Design review of the part shown in the three views and the two pictorial views. Dimensions are in mm from the part's minimum x, y and z. A direction names the side the tool comes from. Give positions to 0.01 mm unless a question says otherwise; leave off trailing zeros. Loops run counter-clockwise (first coordinate to the right, second up) from the corner with the lowest first, then second, coordinate; pieces in that order, holes last. Notation, with made-up numbers: (62, 25.5) - (71, 25.5) arc R20 cw to (71, 37.5) - close; hole circle Ø6 at (40.25, 3). An arc over 180 degrees is marked (long way). Put each result on its own line as item: value. Start each with the question number.
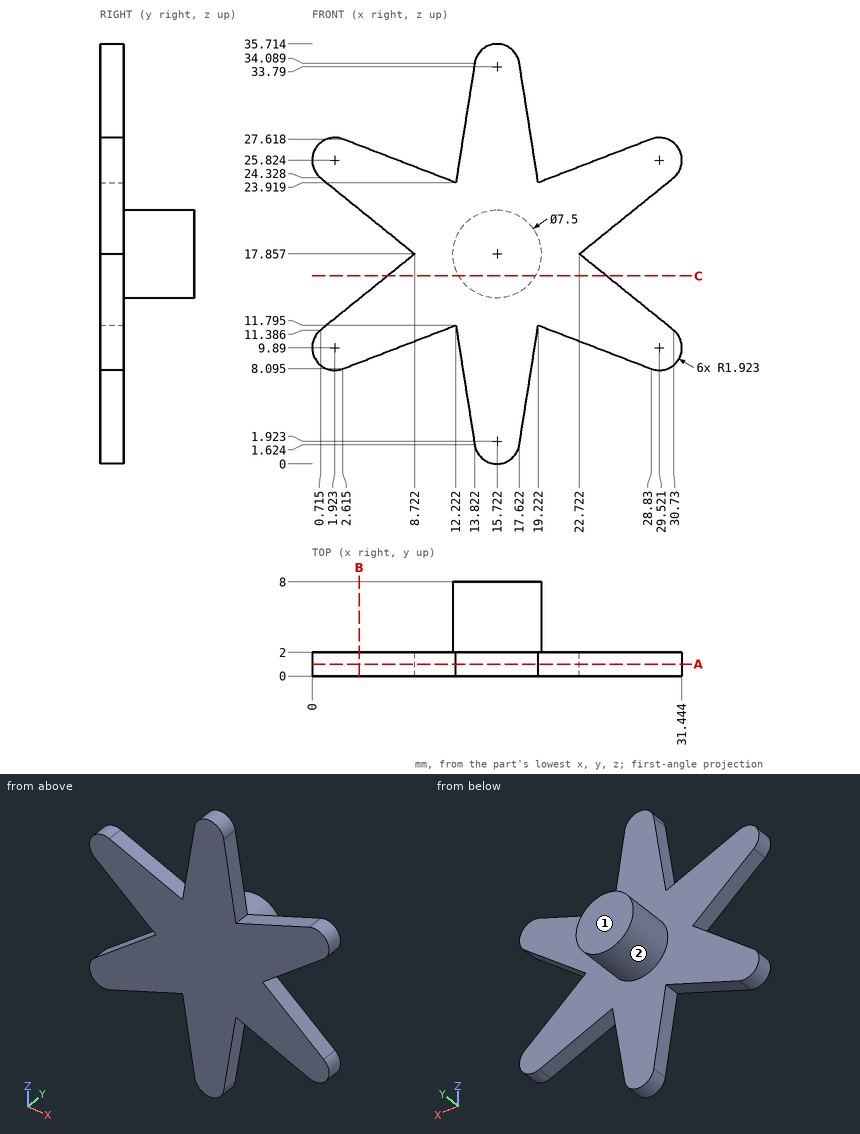
1) Take a section at A-A on y = 1. State the section outline as (x, z) points (1 decimal).
2) Machinability: for the marked faces 1 and 2, which of the approach directions +Z, -Z, +X, -X, +Y, -Y give a long, thin tool a straight path to every point of the face, cutting with its end or side? Answer none if there is none.
3) Take a section at C-C on z = 16. State the section outline as (x, y) points (1 decimal).
4) Wall thickness on probe 1 along Y at (x, z) = (13, 15); probe 2 along Z at (x, y) = (6, 0.5) (1 decimal); probe 3 along Z at (x, y) = (13.5, 7) (1 decimal): over which ranges is each line inside the solid? List them lowest first.
5) Insertion check: P1, Ø8, axis at x = 5.5, z = 32, coming from the -Y side; P2, Ø9.5, axis at x = 13, z = 26, coming from the +Y side. Each pin has a flat end and moves straight along its axis. Give the tip position at first contact, or say it passes through.
6) Take a section at B-B on x = 4. State the section outline as (y, z) points (1 decimal).
Answers follow:
1. outline: (0.7, 11.4) arc R1.9 ccw to (2.6, 8.1) - (12.2, 11.8) - (13.8, 1.6) arc R1.9 ccw to (17.6, 1.6) - (19.2, 11.8) - (28.8, 8.1) arc R1.9 ccw to (30.7, 11.4) - (22.7, 17.9) - (30.7, 24.3) arc R1.9 ccw to (28.8, 27.6) - (19.2, 23.9) - (17.6, 34.1) arc R1.9 ccw to (13.8, 34.1) - (12.2, 23.9) - (2.6, 27.6) arc R1.9 ccw to (0.7, 24.3) - (8.7, 17.9) - close
2. face 1: +Z, -Z, +X, -X, +Y
2. face 2: +Y
3. outline: (6.4, 0) - (25, 0) - (25, 2) - (19, 2) - (19, 8) - (12.5, 8) - (12.5, 2) - (6.4, 2) - close
4. probe 1: 0 to 2
4. probe 2: 9.4 to 15.7, 20.1 to 26.3
4. probe 3: 14.8 to 20.9
5. P1: through
5. P2: y = 2
6. outline: (0, 8.6) - (2, 8.6) - (2, 14) - (0, 14) - close; (0, 21.7) - (2, 21.7) - (2, 27.1) - (0, 27.1) - close
